CAD build for the part. Positions are in the model's coordinates, mm. A direction names the side the tool comes from. Round coordinates to 2 decimals unless told otherwise and drop trailing zeros. Order: outer loops, then holes, each group sorted by start corner. A loop starts at its lowest first (then second) coordinate and runs counter-clockwise, first axis right, second up. Notation, with made-up numbers: M 81.5,-31 L 101.5,-31 A24 cw 101.5,-11 Z; hole C 21,52.5 d7. An arc over 180 degrees is marked long. Answer as a JSON object with one key per item and string values. Group by question number.
Autodesk Fusion 360 part; units mm, degrees
sketch "Sketch1" plane through (0, 0, 0) normal (0, 0, 1) x (1, 0, 0)
  line L0 (-50, 25) -> (-2.5, 25)
  line L1 (-2.5, 25) -> (-2.5, -6)
  line L2 (-2.5, -6) -> (-50, -6)
  line L3 (-50, -6) -> (-50, 25)
  circle A0 centre (-45, 20) radius 1
  circle A1 centre (-32.5, 20) radius 1
  circle A2 centre (-45, -1) radius 1
  circle A3 centre (-32.5, -1) radius 1
  dimension "d1" = 2
  dimension "d2" = 2
  dimension "d3" = 2
  dimension "d4" = 2
  dimension "d5" = 12.5
  dimension "d6" = 5
  dimension "d7" = 5
  dimension "d8" = 12.5
  dimension "d9" = 21
  dimension "d10" = 21
  dimension "d11" = 5
  dimension "d12" = 5
  dimension "d13" = 5
  dimension "d14" = 5
  dimension "d15" = 30
  dimension "d16" = 47.5
  dimension "d17" = 31
extrude "Extrude1" add sketch "Sketch1" along normal blind 3
sketch "Sketch2" plane through (0, 0, 3) normal (0, 0, 1) x (-1, 0, 0)
  circle A0 centre (45, 1) radius 1
  circle A1 centre (32.5, 1) radius 1
  circle A2 centre (32.5, -20) radius 1
  circle A3 centre (45, -20) radius 1
  line L0 (50, 6) -> (2.5, 6)
  line L1 (2.5, 6) -> (2.5, -25)
  line L2 (2.5, -25) -> (50, -25)
  line L3 (50, -25) -> (50, 6)
  line L4 (2.5, -25) -> (5.5, -25)
  line L5 (5.5, -25) -> (5.5, 6)
  line L6 (5.5, 6) -> (2.5, 6)
  line L7 (2.5, 6) -> (2.5, -25)
  dimension "d20" = 3
  dimension "d21" = 31
extrude "Extrude2" add sketch "Sketch2" along normal blind 44.5 contours L0 L1 L2 L4 L5 L6 L7
sketch "Sketch3" plane through (-5.5, 0, 0) normal (-1, 0, 0) x (0, -1, 0)
  line L0 (-25, 3) -> (6, 3)
  line L1 (6, 3) -> (6, 47.5)
  line L2 (6, 47.5) -> (-25, 47.5)
  line L3 (-25, 47.5) -> (-25, 3)
  circle A0 centre (-20, 42.5) radius 1.25
  circle A1 centre (1, 42.5) radius 1.25
  circle A2 centre (-20, 8) radius 1.25
  circle A3 centre (1, 8) radius 1.25
  dimension "d24" = 2.5
  dimension "d25" = 2.5
  dimension "d26" = 2.5
  dimension "d27" = 2.5
  dimension "d28" = 5
  dimension "d29" = 5
  dimension "d30" = 5
  dimension "d31" = 5
  dimension "d32" = 5
  dimension "d33" = 5
  dimension "d34" = 5
  dimension "d35" = 5
extrude "Extrude3" cut sketch "Sketch3" against normal blind 3 contours A0 | A1 | A2 | A3
Item 1: Flat gauge pins, fed straight in: pin 1 Ø10 at (y, z) = (21.5, 17) entering from -X; pin 2 Ø3 at (y, z) = (20, 8) entering from +X; pin 3 Ø1.2 at (x, y) = (-45, 20) entering from -Z; pin 4 Ø2.5 at (x, y) = (-45, -1) entering from +Z. Where does each tip first touch, or does it go through?
Item 2: Drill centre lines: line 1 (Y direction, x = -45, z = 1); line 2 (Z direction, x = -4, y = 20); line 3 (Y direction, x = -3, z = 42). Where is each one in solid material? Low to high. Write a range as [from, to].
Item 3: Two-plate mould, pull along X, no slides. Class faces 3 (the face through (-44, 20, 1)), 4 (the face through (-4, 9, 47.5)), 5 (the face through (-32.717, 20.976, 1.479)), 6 (the face through (-2.5, 10, 23)): +X half, -X half, draft (parallel to the pull), parting line (faces both ways), or undercut.
Item 4: 3-axis set-ups, long thin cutter, end or side, ignore diameter. For faces 1 (the face through (-27, 10, 0)), 2 (the face through (-5.5, 10, 25)): which of +Z, -Z, +X, -X, +Y, -Y reach the whole face in a straight line?
Item 5: Cut at C-C, the plane x = -45. Give the cut face in (y, z), and give its area (3 significant figures).
Item 6: Cut at B-B, the plane z = 42.5. Give the cut face in (x, y), and give its area (3 significant figures).
Item 7: Cut at A-A, the plane y = -1. Give the cut face in (x, z).
Item 8: Cut at D-D, the plane y = 2.5. Give the cut face in (x, z), and give its area (3 significant figures).
Response values:
{
 "1": {"pin 1": "x = -5.5", "pin 2": "x = -2.5", "pin 3": "through", "pin 4": "z = 3"},
 "2": {"line 1": "[-6, -2], [0, 19], [21, 25]", "line 2": "[0, 6.75], [9.25, 41.25], [43.75, 47.5]", "line 3": "[-6, -2.15], [0.15, 18.85], [21.15, 25]"},
 "3": {"face 3": "undercut", "face 4": "draft", "face 5": "undercut", "face 6": "+X half"},
 "4": {"face 1": "-Z, +X, -X, +Y, -Y", "face 2": "+Z, -X, +Y, -Y"},
 "5": {"outline": "M -6,0 L -2,0 L -2,3 L -6,3 Z; M 0,0 L 19,0 L 19,3 L 0,3 Z; M 21,0 L 25,0 L 25,3 L 21,3 Z", "area": "81.0 mm^2"},
 "6": {"outline": "M -5.5,-6 L -2.5,-6 L -2.5,-2.25 L -5.5,-2.25 Z; M -5.5,0.25 L -2.5,0.25 L -2.5,18.75 L -5.5,18.75 Z; M -5.5,21.25 L -2.5,21.25 L -2.5,25 L -5.5,25 Z", "area": "78.0 mm^2"},
 "7": {"outline": "M -50,0 L -46,0 L -46,3 L -50,3 Z; M -44,0 L -33.5,0 L -33.5,3 L -44,3 Z; M -31.5,0 L -2.5,0 L -2.5,6.75 L -5.5,6.75 L -5.5,3 L -31.5,3 Z; M -5.5,9.25 L -2.5,9.25 L -2.5,41.25 L -5.5,41.25 Z; M -5.5,43.75 L -2.5,43.75 L -2.5,47.5 L -5.5,47.5 Z"},
 "8": {"outline": "M -50,0 L -2.5,0 L -2.5,47.5 L -5.5,47.5 L -5.5,3 L -50,3 Z", "area": "276 mm^2"}
}
